```python
from build123d import *

# Parameters (mm, degrees)
F0_W     = 152.4
F0_H     = 76.2
F1_DEPTH = 1981.2
F2_W     = 1524
F2_H     = 762
F2_W_2   = 59.057254
F3_DEPTH = 711.2


with BuildPart() as f1:
    # F0 (on Right) → F1 (new body)
    with BuildSketch(Plane.YZ):
        with BuildLine():
            Line((208.894142, 713.451522), (-349.905858, 713.451522))
            Line((-349.905858, 713.451522), (-349.905858, -200.948478))
            Line((-349.905858, -200.948478), (-195.334996, -200.948478))
            ThreePointArc((-195.334996, -200.948478), (5.694142, 0.080659), (206.723279, -200.948478))
            Line((206.723279, -200.948478), (361.294142, -200.948478))
            Line((361.294142, -200.948478), (361.294142, 713.451522))
            Line((361.294142, 713.451522), (208.894142, 713.451522))
        make_face()
        with Locations((285.094142, 751.551522)):
            Rectangle(F0_W, F0_H)
    extrude(amount=F1_DEPTH)

    # F2 (on face) → F3 (cut)
    with BuildSketch(Plane.XZ.offset(349.905858)):
        with Locations((762, 180.051522)):
            Rectangle(F2_W, F2_H)
        with Locations((-29.528627, 180.051522)):
            Rectangle(F2_W_2, F2_H)
    extrude(amount=-F3_DEPTH, mode=Mode.SUBTRACT)


solid = f1.part
```
Work out the finished part from the listing and answer in its coordinate system (mm). A direction names the side the tool comes from. Give positions to 0.01 mm unless a question says otherwise; leave off trailing zeros. Order: outer loops, then holes, each group sorted by start corner. A loop starts at its lowest first (then second) coordinate and runs counter-clockwise, first axis right, second up.
1. Straight lines are drawn through the part: L1, parallel to Z at x = 1339.5, y = 120; L2, parallel to X at y = 123, z = 260; L3, parallel to Z at x = 635, y = 332.5. For each, find the intervals that lie inside material, in ascending order.
Result sheet:
L1: z = 561.05 to 713.45
L2: x = 1524 to 1981.2
L3: z = 561.05 to 789.65
2. Section B-B, the plane x = 1726 is taken. Determine the outline of the cut face in (y, z) (3 decimals), and give its area (3 significant figures).
Result sheet:
outline: (-349.906, -200.948) - (-195.335, -200.948) arc R201.029 cw to (206.723, -200.948) - (361.294, -200.948) - (361.294, 789.652) - (208.894, 789.652) - (208.894, 713.452) - (-349.906, 713.452) - close
area: 598,000 mm2
3. Each of these flat-tipped pins is pushed along its axis until it touches: P1, Ø10, axis at x = 794, y = -9.5, coming from the +Z side; P2, Ø10, axis at y = 32, z = 49.5, coming from the -X side; P3, Ø3, axis at x = 1330, y = 226.5, coming from the -Z side. Where does it stop, or does it pass through?
Result sheet:
P1: stops at z = 713.45
P2: stops at x = 1524
P3: stops at z = 561.05
4. The mould has two halves that part along Y. Classify faces 1 (the flat face through (977, 208.894, 751)), 2 (the cylindrical face through (1749.4, 1.27, 0.03)), 3 (the flat face through (773, 1, 561.052)): released by +Y, released by -Y, zero draft, split by the parting line, or undercut.
Result sheet:
face 1: released by -Y
face 2: undercut
face 3: zero draft
5. For faces 4 (the flat face through (1524, 1, 175)), 5 (the flat face through (1981.2, 1, 301)), 6 (the flat face through (977, -67, 713.452)), determine the directions among +Z, -Z, +X, -X, +Y, -Y from which every point of the face is accessible in a straight line to the end or side of a thin tool.
Result sheet:
face 4: -Z, -X, +Y, -Y
face 5: +Z, -Z, +X, +Y, -Y
face 6: +Z, +X, -X, -Y
6. Section C-C, the plane z = 370.5 is taken. Determine the outline of the cut face in (x, y), and give its area (3 significant figures).
Result sheet:
outline: (1524, -349.91) - (1981.2, -349.91) - (1981.2, 361.29) - (1524, 361.29) - close
area: 325,000 mm2
7. Section A-A, the plane y = -275 is taken. Determine the outline of the cut face in (x, z).
Result sheet:
outline: (0, 561.05) - (1524, 561.05) - (1524, -200.95) - (1981.2, -200.95) - (1981.2, 713.45) - (0, 713.45) - close
8. Section D-D, the plane y = 248.5 is taken. Determine the outline of the cut face in (x, z).
Result sheet:
outline: (0, 561.05) - (1524, 561.05) - (1524, -200.95) - (1981.2, -200.95) - (1981.2, 789.65) - (0, 789.65) - close
